```python
from build123d import *

# Parameters (mm, degrees)
BOSS_EXTRUDE1_DEPTH = 6.35


with BuildPart() as part:
    # Sketch1 → Boss-Extrude1 (new body)
    with BuildSketch(Plane(origin=(0, 0, 0), x_dir=(1, 0, 0), z_dir=(0, 1, 0))):
        with BuildLine():
            Line((71.12, 4.935349186), (71.12, -22.938860698))
            Line((71.12, -22.938860698), (54.725773369, -12.242694437))
            Line((54.725773369, -12.242694437), (0.106224527, -12.699555754))
            ThreePointArc((0.106224527, -12.699555754), (-0.64393835, -12.683664431), (-1.391853504, -12.623499666))
            Line((-1.391853504, -12.623499666), (-71.12, -4.935349186))
            Line((-71.12, -4.935349186), (-71.12, 22.938860698))
            Line((-71.12, 22.938860698), (-54.725773369, 12.242694437))
            Line((-54.725773369, 12.242694437), (-0.106224527, 12.699555754))
            ThreePointArc((-0.106224527, 12.699555754), (0.64393835, 12.683664431), (1.391853504, 12.623499666))
            Line((1.391853504, 12.623499666), (71.12, 4.935349186))
        make_face()
        with BuildLine():
            Line((-2.5527, 1.734282538), (-2.5527, -1.734282538))
            ThreePointArc((-2.5527, -1.734282538), (3.0861, 0), (-2.5527, 1.734282538))
        make_face(mode=Mode.SUBTRACT)
    extrude(amount=BOSS_EXTRUDE1_DEPTH)


solid = part.part
```
Source: CAD feature listing. Evaluate the final solid. Frame: model axes, mm. Coordinates: 2 decimals unless noted, no trailing zeros. Loops run counter-clockwise (first coordinate to the right, second up) from the corner with the lowest first, then second, coordinate; pieces in that order, holes last. Notation, with made-up numbers: M 28.25,49 L 76.25,49 A6 cw 76.25,59 Z; hole C 27.25,80 d5. An arc over 180 degrees is marked long. Put each result on its own line as item: value. Start each with the question number.
1) Pull-direction query (X, two-part tool) for faces 1 (the face through (35.768, 3.131, -8.833)), 2 (the face through (1, 0, -5)), 3 (the face through (-2.553, 3, 0)); classes: pulls with the +X half, pulls with the -X half, needs draft (parallel to the pull), parting line crosses it, or undercut.
2) Contact query for flat-ended pins moving along their axis: pin 1 Ø2 at (x, z) = (-48, -10) entering from -Y; pin 2 Ø1 at (x, y) = (8, 5.5) entering from -Z; pin 3 Ø1 at (x, y) = (17.5, 1.5) entering from -Z; pin 4 Ø10 at (x, z) = (-47.5, -18) entering from -Y. Output: stop coordinate, or through.
3) Cut plane B-B on x = 46. Return the cut outline in (y, z).
4) Cut plane C-C on z = -16. Return the cut outline in (x, y), then the cut area to 3 significant figures.
5) Ray query, L1, parallel to X at y = 4.75, z = 0; L2, parallel to Z at x = 0, y = 2.5; L3, parallel to X at y = 5, z = 13.5. Return the intervals inside material, ascending. Write a range as from..to.
6) Cut plane A-A on z = 0. Return the cut outline in (x, y).
The answers:
1. face 1: pulls with the +X half
1. face 2: needs draft
1. face 3: undercut
2. pin 1: stops at y = 0
2. pin 2: stops at z = -11.95
2. pin 3: stops at z = -10.9
2. pin 4: passes through
3. outline: M 0,-7.71 L 6.35,-7.71 L 6.35,12.32 L 0,12.32 Z
4. outline: M -71.12,0 L -60.48,0 L -60.48,6.35 L -71.12,6.35 Z
4. area: 67.5 mm²
5. L1: x = -71.12..-2.55, 3.09..71.12
5. L2: z = -12.7..-3.09, 3.09..12.7
5. L3: x = 56.65..71.12
6. outline: M -71.12,0 L -2.55,0 L -2.55,6.35 L -71.12,6.35 Z; M 3.09,0 L 71.12,0 L 71.12,6.35 L 3.09,6.35 Z
